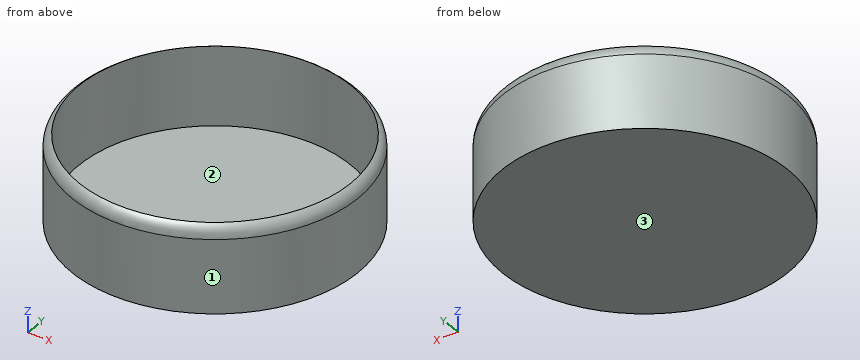
from build123d import *

# Parameters (mm, degrees)
F0_R     = 50
F1_DEPTH = 30
F2_T     = -2.5


# Not quite as in the source:
# - a fillet or chamfer that OpenCascade refuses, or shapes differently, is made with other operations: its cross-section is extruded or revolved along the edge and cut away or added


with BuildPart() as f1:
    # F0 (on Top) → F1 (new body)
    with BuildSketch(Plane.XY):
        Circle(F0_R)
    extrude(amount=F1_DEPTH)

    # F2
    f2_openings = [f1.faces().sort_by_distance(p)[0] for p in [
        (0, 0, 30),
    ]]
    offset(amount=F2_T, openings=f2_openings)

    # F3: fillet of radius 5 on 1 edges, made by hand

    # F3_s1 → F3_t2 (revolve, cut)
    with BuildSketch(Plane.XZ):
        with BuildLine():
            ThreePointArc((50, 25.6698729811), (49.3301270189, 28.1698729811), (47.5, 30))
            Line((47.5, 30), (50, 30))
            Line((50, 30), (50, 25.6698729811))
        make_face()
    revolve(axis=Axis((0, 0, 30), (0, 0, 1)), mode=Mode.SUBTRACT)


solid = f1.part
The listing builds one solid part. Answer for the finished solid, in the listing's coordinates (mm). Face numbers are marked on the shaded views. Give positions to 0.01 mm unless a question says otherwise; leave off trailing zeros. Write each loop counter-clockwise with the first axis right and the second up, starting at its lowest first coordinate (ties: lowest second). Pieces come first, ordered by that corner, then holes. Notation, with made-up numbers: (-21.75, 29) -> (-1.75, 29) arc R28 cw to (-1.75, 55) -> close; hole circle Ø8 at (4, 81). An arc over 180 degrees is marked (long way). Use a Markdown table: item, result.
(1) Find the intervals of material crossed by probe 1 along Y at (x, z) = (0, 11.75); probe 2 along Z at (x, y) = (18, -3); probe 3 along Y at (x, z) = (41, 21), in increasing order. Write a range as from..to.
Return value:
| item | result |
|---|---|
| probe 1 | -50..-47.5, 47.5..50 |
| probe 2 | 0..2.5 |
| probe 3 | -28.62..-23.98, 23.98..28.62 |
(2) Section D-D, the plane z = 27.25 is taken. Determine the outline of the cut face in (x, y).
Return value:
| item | result |
|---|---|
| outline | circle Ø99.49 at (0, 0); hole circle Ø95 at (0, 0) |
(3) Flat-ended cylindrical pins translate along their axes: P1, Ø5, axis at x = -32, z = 3.5, coming from the -Y side; P2, Ø4, axis at x = 8, z = 26, coming from the +Y side; P3, Ø1, axis at y = -16.5, z = 17, coming from the -X side. Find the tip coordinate at first contact, or state that the pin passes through.
Return value:
| item | result |
|---|---|
| P1 | y = -40.37 |
| P2 | y = 49.64 |
| P3 | x = -47.37 |
(4) Section B-B, the plane z = 13.5 is taken. Determine the outline of the cut face in (x, y), then the cut area to 3 significant figures.
Return value:
| item | result |
|---|---|
| outline | circle Ø100 at (0, 0); hole circle Ø95 at (0, 0) |
| area | 766 mm2 |
(5) Section A-A, the plane x = 0 is taken. Determine the outline of the cut face in (y, z).
Return value:
| item | result |
|---|---|
| outline | (-50, 0) -> (50, 0) -> (50, 25.67) arc R5 ccw to (47.5, 30) -> (47.5, 2.5) -> (-47.5, 2.5) -> (-47.5, 30) arc R5 ccw to (-50, 25.67) -> close |
(6) Determine the mould class of the marked faces 1, 2 and 3 for opening direction X: released by +X, released by -X, zero draft, split by the parting line, or undercut.
Return value:
| item | result |
|---|---|
| face 1 | split by the parting line |
| face 2 | undercut |
| face 3 | zero draft |
